Input: part model. Units: mm. Frame: model coordinates. A direction names the side the tool comes from. Coordinates: 2 decimals unless noted, no trailing zeros. Write each loop counter-clockwise with the first axis right and the second up, starting at its lowest first coordinate (ties: lowest second). Pieces come first, ordered by that corner, then holes.
1) Line query: L1, parallel to Z at x = 1, y = 4.5; L2, parallel to X at y = 1.25, z = -2; L3, parallel to Z at x = -0.75, y = -0.75. Output: solid intervals per line, ascending.
2) Set-up query: faces 1 (the flat face through (1.293, -1.776, -0.76)), 2 (the flat face through (0, 16, 0)). Return all of +Z, -Z, +X, -X, +Y, -Y with unobstructed straight access to the full face (end or side cutting, diameter ignored); none if empty.
3) Pin query (flat end, axial travel): pin 1 Ø4 at (x, y) = (-3, -0.5) entering from +Z; pin 2 Ø0.5 at (x, y) = (0.5, -2) entering from +Z; pin 3 Ø2 at (y, z) = (9, 3) entering from +X. Return the tip coordinate at first contact, or that it passes through.
4) Draft query along X for faces 3 (the flat face through (2.04, 0, 2.04)), 4 (the flat face through (-1.293, -1.776, 0.76)), 5 (the cylindrical face through (-0.54, 8.04, 2.44)). Return one class per face: pulls with the +X half, pulls with the -X half, needs draft (parallel to the pull), parting line crosses it, or undercut.
5) Section query A-A (y = 14). Output: boundary loops of the cut face in (x, z), then the cut area to 3 significant figures.
Solid Edge part; units mm, degrees
sketch "Sketch1" plane through (0, 0, 0) normal (0, 0, 1) x (1, 0, 0)
  line L0 (2.5, 0) -> (2.5, 16)
  line L1 (0, 16) -> (2.5, 16)
  line L2 (0, 0) -> (0, 16)
  line L3 (0, 0) -> (0, -2.75)
  line L4 (0, -2.75) -> (4.75, -2.75)
  line L5 (4.75, -2.75) -> (4.75, 0)
  line L6 (4.75, 0) -> (2.5, 0)
revolve "RevolvedProtrusion1" add sketch "Sketch1" angle 360 about axis through (0, 0, 0) along (0, 1, 0)
sketch "Sketch2" plane through (0, 0, 0) normal (1, 0, 0) x (0, 1, 0)
  line L0 (-2.75, 2.2215) -> (-1.19, 2.2215)
  line L1 (0.0926, 0) -> (-1.19, 2.2215)
  line L2 (-2.75, 0) -> (0.0926, 0)
  line L3 (-2.75, 0) -> (-2.75, 2.2215)
revolve "RevolvedCutout1" cut sketch "Sketch2" angle 360 about axis through (0, -4.5, 0) along (0, 1, 0)
sketch "Sketch3" plane through (0, -2.75, 0) normal (0, -1, 0) x (0, 0, 1)
  circle A0 centre (0, 0) radius 2.2215
  line L0 (-1.5, -0.866) -> (0, -1.7321)
  line L1 (0, -1.7321) -> (1.5, -0.866)
  line L2 (1.5, -0.866) -> (1.5, 0.866)
  line L3 (1.5, 0.866) -> (0, 1.7321)
  line L4 (0, 1.7321) -> (-1.5, 0.866)
  line L5 (-1.5, 0.866) -> (-1.5, -0.866)
extrude "Protrusion1" add sketch "Sketch3" against normal up to next
sketch "Sketch4" plane through (0, 0, 0) normal (0, 0, 1) x (1, 0, 0)
  line L0 (-1.7321, -2.75) -> (0, -2.75)
  line L1 (0, -2.75) -> (0, -2.2859)
  line L2 (0, -2.2859) -> (-1.7321, -2.75)
revolve "RevolvedCutout2" cut sketch "Sketch4" angle 360 about axis through (0, -4.5, 0) along (0, 1, 0)
fillet "Round1" radius 0.2 1 edges at (0, 0, -2.5)
chamfer "倒斜角_2" distance 0.3333 angle 45 1 edges at (0, 16, -2.5)
cosmetic_thread "螺纹_3" thread depth 14.4
sketch "Sketch5" plane through (0, 0, 0) normal (0, 0, 1) x (1, 0, 0)
  arc A0 (-2.2953, -2.75) -> (-4.75, 0) centre (-1.9822, 0) cw
revolve "RevolvedCutout3" cut sketch "Sketch5" angle 360 about axis through (0, 0, 0) along (0, -1, 0) material side at (-4.0844, -1.8764, 0)
Answer:
1. L1: z = -2.29 to 2.29
1. L2: x = -1.5 to 1.5
1. L3: z = -4.59 to -1.25, 1.25 to 4.59
2. face 1: -Y
2. face 2: +Z, -Z, +X, -X, +Y
3. pin 1: stops at z = 4.63
3. pin 2: stops at z = 4.1
3. pin 3: stops at x = 1.5
4. face 3: needs draft
4. face 4: undercut
4. face 5: parting line crosses it
5. outline: circle Ø5 at (0, 0)
5. area: 19.6 mm2
